Check sheet for the modelled part. Datum: model origin and axes. Units: mm. A direction names the side the tool comes from. Coordinates: 2 decimals unless noted, no trailing zeros. Loops run counter-clockwise (first coordinate to the right, second up) from the corner with the lowest first, then second, coordinate; pieces in that order, holes last. Notation, with made-up numbers: (78.5, 35.5) -> (106.5, 35.5) arc R7 cw to (106.5, 44.5) -> close; hole circle Ø10 at (-29, 77.5). An arc over 180 degrees is marked (long way). Use CSV: the item, a comma, the result in double quotes. Start each with the question number.
1. Release check for a two-part mould opening along X. For faces 4 (the face through (37.088, -18, 1)), 5 (the face through (3, -18, 0)), 6 (the face through (3, -26.67, 1)) record: pulls with the +X half, pulls with the -X half, needs draft (parallel to the pull), parting line crosses it, or undercut.
2. Thickness scan on L1, parallel to X at y = -11.5, z = -35.5; L2, parallel to Y at x = 9.5, z = -14.5; L3, parallel to Z at x = 7, y = -41. Record the ranges inside material, lowest first.
3. Set-up check for faces 1 (the face through (-30.976, -18, 2)), 2 (the face through (3, -10.414, -19)), 3 (the face through (3, -36, 8.473)): record each of +Z, -Z, +X, -X, +Y, -Y from which the full face is reachable in a straight line by a thin tool's end or side.
4. Sectioned sample at A-A, the plane z = -32. Record the cut outline in (x, y).
5. Gauge pin test, flat ends, axial feed: pin 1 (4 mm diameter, centred on x = -14, z = -16, fed in from +Y); pin 2 (5 mm diameter, centred on x = 11, y = -18.5, fed in from -Z); pin 3 (23.5 mm diameter, centred on x = -11, z = -11, fed in from -Y). Record the tip position at first contact, or that the pin passes through.
6. Sectioned sample at D-D, the plane x = -24.5. Record the cut outline in (y, z), and give its area (3 significant figures).
7. Sectioned sample at C-C, the plane y = -33. Record the cut outline in (x, z), and give its area (3 significant figures).
8. Sectioned sample at B-B, the plane x = 5.5. Record the cut outline in (y, z), and give its area (3 significant figures).
```python
from build123d import *

# Parameters (mm, degrees)
F0_W     = 68.0640637875
F0_H     = 65.563749522
F1_DEPTH = 26.67
F2_W     = 36.6712510586
F2_H     = 47.2281239927
F3_DEPTH = 16.256
F5_DEPTH = 19.304
F6_W     = 36.6712510586
F6_H     = 8.4732808173
F7_DEPTH = 16.256


with BuildPart() as f1:
    # F0 (on Front) → F1 (new body)
    with BuildSketch(Plane.XZ):
        with Locations((3.0559375882, -5.9729684144)):
            Rectangle(F0_W, F0_H)
    extrude(amount=F1_DEPTH)

    # F2 (on face) → F3 (cut)
    with BuildSketch(Plane.XZ.offset(26.67)):
        with Locations((3.1948443502, -15.1407811791)):
            Rectangle(F2_W, F2_H)
    extrude(amount=-F3_DEPTH, mode=Mode.SUBTRACT)

    # F4 (on face) → F5 (join)
    with BuildSketch(Plane.XZ.offset(26.67)):
        Polygon((37.0879694819, 26.8089063466), (-30.9760943055, 26.8089063466), (-30.9760943055, 8.4732808173), (-15.1407811791, 8.4732808173), (21.5304698795, 8.4732808173), (37.0879694819, 8.4732808173), align=None)
    extrude(amount=F5_DEPTH)

    # F6 (on face) → F7 (join)
    with BuildSketch(Plane.XZ.offset(10.414)):
        with Locations((3.1948443502, 4.2366404086)):
            Rectangle(F6_W, F6_H)
    extrude(amount=F7_DEPTH)


solid = f1.part
```
Completed:
1,face 4,"pulls with the +X half"
1,face 5,"undercut"
1,face 6,"needs draft"
2,L1,"-30.98 to -15.14, 21.53 to 37.09"
2,L2,"-10.41 to 0"
2,L3,"8.47 to 26.81"
3,face 1,"+Z, -Z, -X, +Y, -Y"
3,face 2,"-Z, -Y"
3,face 3,"-Z, +X, -X, -Y"
4,outline,"(-30.98, -26.67) -> (-15.14, -26.67) -> (-15.14, -10.41) -> (21.53, -10.41) -> (21.53, -26.67) -> (37.09, -26.67) -> (37.09, 0) -> (-30.98, 0) -> close"
5,pin 1,"y = 0"
5,pin 2,"z = 0"
5,pin 3,"y = -26.67"
6,outline,"(-45.97, 8.47) -> (-26.67, 8.47) -> (-26.67, -38.75) -> (0, -38.75) -> (0, 26.81) -> (-45.97, 26.81) -> close"
6,area,"2,100 mm²"
7,outline,"(-30.98, 8.47) -> (37.09, 8.47) -> (37.09, 26.81) -> (-30.98, 26.81) -> close"
7,area,"1,250 mm²"
8,outline,"(-45.97, 8.47) -> (-26.67, 8.47) -> (-26.67, 0) -> (-10.41, 0) -> (-10.41, -38.75) -> (0, -38.75) -> (0, 26.81) -> (-45.97, 26.81) -> close"
8,area,"1,470 mm²"
